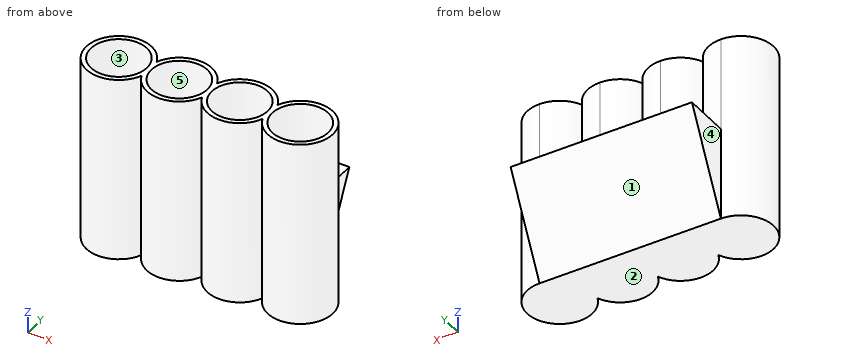
```python
from build123d import *

# Parameters (mm, degrees)
F0_R     = 7.62
F1_DEPTH = 50.8
F2_DEPTH = 25.4
F4_DEPTH = 61.468
F5_DEPTH = 2.54


with BuildPart() as f1:
    # F0 (on Top) → F1 (new body)
    with BuildSketch(Plane.XY):
        with BuildLine():
            ThreePointArc((16.51, 8.89), (11.525071, 7.360882), (8.255, 3.299557))
            ThreePointArc((8.255, 3.299557), (4.984929, 7.360882), (0, 8.89))
            ThreePointArc((0, 8.89), (-7.360882, -4.984929), (8.255, -3.299557))
            ThreePointArc((8.255, -3.299557), (16.51, -8.89), (24.765, -3.299557))
            ThreePointArc((24.765, -3.299557), (33.02, -8.89), (41.275, -3.299557))
            ThreePointArc((41.275, -3.299557), (56.890882, -4.984929), (49.53, 8.89))
            ThreePointArc((49.53, 8.89), (44.545071, 7.360882), (41.275, 3.299557))
            ThreePointArc((41.275, 3.299557), (38.004929, 7.360882), (33.02, 8.89))
            ThreePointArc((33.02, 8.89), (28.035071, 7.360882), (24.765, 3.299557))
            ThreePointArc((24.765, 3.299557), (21.494929, 7.360882), (16.51, 8.89))
        make_face()
        Circle(F0_R, mode=Mode.SUBTRACT)
        with Locations((16.51, 0)):
            Circle(F0_R, mode=Mode.SUBTRACT)
        with Locations((33.02, 0)):
            Circle(F0_R, mode=Mode.SUBTRACT)
        with Locations((49.53, 0)):
            Circle(F0_R, mode=Mode.SUBTRACT)
    extrude(amount=F1_DEPTH)

    # F0 (on Top) → F2 (join)
    with BuildSketch(Plane.XY):
        with BuildLine():
            Line((49.53, 8.89), (33.02, 8.89))
            ThreePointArc((33.02, 8.89), (38.004929, 7.360882), (41.275, 3.299557))
            ThreePointArc((41.275, 3.299557), (44.545071, 7.360882), (49.53, 8.89))
        make_face()
        with BuildLine():
            Line((33.02, 8.89), (16.51, 8.89))
            ThreePointArc((16.51, 8.89), (21.494929, 7.360882), (24.765, 3.299557))
            ThreePointArc((24.765, 3.299557), (28.035071, 7.360882), (33.02, 8.89))
        make_face()
        with BuildLine():
            ThreePointArc((0, 8.89), (4.984929, 7.360882), (8.255, 3.299557))
            ThreePointArc((8.255, 3.299557), (11.525071, 7.360882), (16.51, 8.89))
            Line((16.51, 8.89), (0, 8.89))
        make_face()
        Polygon((0, 21.59), (0, 8.89), (16.51, 8.89), (33.02, 8.89), (49.53, 8.89), (49.53, 21.59), align=None)
    extrude(amount=F2_DEPTH)

    # F3 (on face) → F4 (cut)
    with BuildSketch(Plane(origin=(0, 0, 0), x_dir=(0, -1, 0), z_dir=(-1, 0, 0))):
        Polygon((-8.89, 0), (-21.59, 25.4), (-21.59, 0), align=None)
    extrude(amount=-F4_DEPTH, mode=Mode.SUBTRACT)

    # F0 (on Top) → F5 (join)
    with BuildSketch(Plane.XY):
        Circle(F0_R)
        with Locations((16.51, 0)):
            Circle(F0_R)
        with Locations((33.02, 0)):
            Circle(F0_R)
        with Locations((49.53, 0)):
            Circle(F0_R)
    extrude(amount=F5_DEPTH)


solid = f1.part
```
Design review of the part built by this model. Coordinates are the model's own, in mm. Face numbers are marked on the shaded views. A direction names the side the tool comes from. Coordinates: 2 decimals unless noted, no trailing zeros. Write each loop counter-clockwise with the first axis right and the second up, starting at its lowest first coordinate (ties: lowest second). Pieces come first, ordered by that corner, then holes. Notation, with made-up numbers: M 64,78 L 87,78 A21 cw 87,94 Z; hole C -13.75,83 d3. An arc over 180 degrees is marked long. Answer as a JSON object with one key per item and string values.
Item 1: Add section D-D, the plane z = 17. Give the boundary of the cut face in (x, y) (3 decimals), and give its area (3 significant figures).
Outcome:
{"outline": "M 0,8.89 A8.89 ccw long 8.255,-3.3 A8.89 ccw 24.765,-3.3 A8.89 ccw 41.275,-3.3 A8.89 ccw long 49.53,8.89 L 49.53,17.39 L 0,17.39 Z; hole C 0,0 d15.24; hole C 16.51,0 d15.24; hole C 33.02,0 d15.24; hole C 49.53,0 d15.24", "area": "744 mm²"}
Item 2: Add section B-B, the plane y = 0. Give the boundary of the cut face in (x, z).
Outcome:
{"outline": "M -8.89,0 L 58.42,0 L 58.42,50.8 L 57.15,50.8 L 57.15,2.54 L 41.91,2.54 L 41.91,50.8 L 40.64,50.8 L 40.64,2.54 L 25.4,2.54 L 25.4,50.8 L 24.13,50.8 L 24.13,2.54 L 8.89,2.54 L 8.89,50.8 L 7.62,50.8 L 7.62,2.54 L -7.62,2.54 L -7.62,50.8 L -8.89,50.8 Z"}
Item 3: Draft analysis for pull direction Y (two halves, no side actions). For the marked faces 1, 2 and 3, state which applies: pulls with the +Y half, pulls with the -Y half, needs draft (parallel to the pull), parting line crosses it, or undercut.
Outcome:
{"face 1": "pulls with the +Y half", "face 2": "needs draft", "face 3": "undercut"}
Item 4: Wall thickness on probe 1 along Y at (x, z) = (0, 36.5); probe 2 along X at (y, z) = (9.5, 23); probe 3 along Z at (x, y) = (51, 3): over which ranges is each line inside the solid? List them lowest first.
Outcome:
{"probe 1": "-8.89 to -7.62, 7.62 to 8.89", "probe 2": "0 to 49.53", "probe 3": "0 to 2.54"}
Item 5: Add section A-A, the plane z = 35. Give the boundary of the cut face in (x, y) (3 decimals), and give its area (3 significant figures).
Outcome:
{"outline": "M 8.255,-3.3 A8.89 ccw 24.765,-3.3 A8.89 ccw 41.275,-3.3 A8.89 ccw long 41.275,3.3 A8.89 ccw 24.765,3.3 A8.89 ccw 8.255,3.3 A8.89 ccw long Z; hole C 0,0 d15.24; hole C 16.51,0 d15.24; hole C 33.02,0 d15.24; hole C 49.53,0 d15.24", "area": "247 mm²"}
Item 6: Machinability: for the marked faces 4 and 5, which of the approach directions +Z, -Z, +X, -X, +Y, -Y give a long, thin tool a straight path to every point of the face, cutting with its end or side? Answer none if there is none.
Outcome:
{"face 4": "+Z, -Z, -X, +Y", "face 5": "+Z"}
Item 7: Insertion check: pin 1 Ø17.5 at (x, y) = (0, 0) entering from +Z; pin 2 Ø4.5 at (x, y) = (15.5, -1) entering from +Z; pin 3 Ø14 at (y, z) = (13.5, 15) entering from +X; pin 4 Ø6.5 at (y, z) = (16.5, 11) entering from -X. Each pin has a flat end and moves straight along its axis. Give the tip position at first contact, or say it passes through.
Outcome:
{"pin 1": "z = 50.8", "pin 2": "z = 2.54", "pin 3": "x = 55.59", "pin 4": "x = 0"}
Item 8: Add section C-C, the plane x = 45.5. Give the boundary of the cut face in (y, z), and give its area (3 significant figures).
Outcome:
{"outline": "M -7.92,0 L 8.89,0 L 21.59,25.4 L 7.92,25.4 L 7.92,50.8 L 6.47,50.8 L 6.47,2.54 L -6.47,2.54 L -6.47,50.8 L -7.92,50.8 Z", "area": "367 mm²"}
